Check sheet for the modelled part. Datum: model origin and axes. Units: mm. A direction names the side the tool comes from. Give positions to 0.01 mm unless a question says otherwise; leave off trailing zeros. Loops run counter-clockwise (first coordinate to the right, second up) from the corner with the lowest first, then second, coordinate; pieces in that order, holes last. Notation, with made-up numbers: (-21.5, 79) -> (11.5, 79) arc R8 cw to (11.5, 90) -> close; hole circle Ø6 at (22.5, 42.5). An arc over 180 degrees is marked (long way). Answer as CSV lines item,"result". Start each with the question number.
(1) Section check C-C on x = 7.5. Enter the section's corners in (y, z), plus the area to 3 significant figures.
(2) Material ranges on line 1 (Y direction, x = -11, z = 8); line 2 (X direction, y = 4.5, z = 4); line 3 (Z direction, x = 16, y = 2.25), recorded low to high. Write a range as from..to.
(3) Release check for a two-part mould opening along Y. For faces 1 (the face through (0, 3, 1)), 2 (the face through (0, -7.5, 27)), 3 (the face through (16.8, -7.64, 26.13)), 4 (the face through (0, 4, 0)) record: pulls with the +Y half, pulls with the -Y half, needs draft (parallel to the pull), parting line crosses it, or undercut.
(4) Gauge pin test, flat end, axial feed: pin 1 Ø4 at (x, y) = (-5.5, 6.5) entering from -Z. Record the tip position at first contact, or that the pin passes through.
(5) Section check D-D on y = 6.5. Enter the section's corners in (x, z).
(6) Section check A-A on z = 7. Enter the section's corners in (x, y), plus the area to 3 significant figures.
(7) Section check B-B on x = 1. Enter the section's corners in (y, z).
(8) Access from +Z, -Z, +X, -X, +Y, -Y to the whole of each face (thin tool, end or side, straight path). Record for faces 5 (the face through (2.2, 2, 0.5)), 6 (the face through (-16.84, -7.6, 26.13)), 7 (the face through (16.7, 0, 27)).
from build123d import *

# Parameters (mm, degrees)
F1_DEPTH = 53
F2_DEPTH = 1
F3_W     = 5
F3_H     = 4
F4_DEPTH = 53.001


with BuildPart() as f1:
    # F0 (on Top) → F1 (new body)
    with BuildSketch(Plane.XY):
        with BuildLine():
            Line((-14.7, -8.5), (14.7, -8.5))
            ThreePointArc((14.7, -8.5), (16.82132, -7.62132), (17.7, -5.5))
            Line((17.7, -5.5), (17.7, 5.5))
            ThreePointArc((17.7, 5.5), (16.82132, 7.62132), (14.7, 8.5))
            Line((14.7, 8.5), (-14.7, 8.5))
            ThreePointArc((-14.7, 8.5), (-16.82132, 7.62132), (-17.7, 5.5))
            Line((-17.7, 5.5), (-17.7, -5.5))
            ThreePointArc((-17.7, -5.5), (-16.82132, -7.62132), (-14.7, -8.5))
        make_face()
        with BuildLine():
            Line((-13.7, 7.5), (13.7, 7.5))
            ThreePointArc((13.7, 7.5), (15.82132, 6.62132), (16.7, 4.5))
            Line((16.7, 4.5), (16.7, -4.5))
            ThreePointArc((16.7, -4.5), (15.82132, -6.62132), (13.7, -7.5))
            Line((13.7, -7.5), (-13.7, -7.5))
            ThreePointArc((-13.7, -7.5), (-15.82132, -6.62132), (-16.7, -4.5))
            Line((-16.7, -4.5), (-16.7, 4.5))
            ThreePointArc((-16.7, 4.5), (-15.82132, 6.62132), (-13.7, 7.5))
        make_face(mode=Mode.SUBTRACT)
    extrude(amount=F1_DEPTH)

    # F0 (on Top) → F2 (join)
    with BuildSketch(Plane.XY):
        with BuildLine():
            ThreePointArc((16.7, 4.5), (15.82132, 6.62132), (13.7, 7.5))
            Line((13.7, 7.5), (-13.7, 7.5))
            ThreePointArc((-13.7, 7.5), (-15.82132, 6.62132), (-16.7, 4.5))
            Line((-16.7, 4.5), (-16.7, -4.5))
            ThreePointArc((-16.7, -4.5), (-15.82132, -6.62132), (-13.7, -7.5))
            Line((-13.7, -7.5), (13.7, -7.5))
            ThreePointArc((13.7, -7.5), (15.82132, -6.62132), (16.7, -4.5))
            Line((16.7, -4.5), (16.7, 4.5))
        make_face()
    extrude(amount=F2_DEPTH)

    # F3 (on face) → F4 (cut, through all)
    with BuildSketch(Plane(origin=(0, 0, 0), x_dir=(1, 0, 0), z_dir=(0, 0, -1))):
        with Locations((2.2, 0)):
            Rectangle(F3_W, F3_H)
    extrude(amount=-F4_DEPTH, mode=Mode.SUBTRACT)


solid = f1.part
Working result:
1,outline,"(-8.5, 0) -> (8.5, 0) -> (8.5, 53) -> (7.5, 53) -> (7.5, 1) -> (-7.5, 1) -> (-7.5, 53) -> (-8.5, 53) -> close"
1,area,"121 mm^2"
2,line 1,"y = -8.5..-7.5, 7.5..8.5"
2,line 2,"x = -17.7..-16.7, 16.7..17.7"
2,line 3,"z = 0..1"
3,face 1,"undercut"
3,face 2,"undercut"
3,face 3,"pulls with the -Y half"
3,face 4,"needs draft"
4,pin 1,"stops at z = 0"
5,outline,"(-17.53, 0) -> (17.53, 0) -> (17.53, 53) -> (15.94, 53) -> (15.94, 1) -> (-15.94, 1) -> (-15.94, 53) -> (-17.53, 53) -> close"
6,outline,"(-17.7, -5.5) arc R3 ccw to (-14.7, -8.5) -> (14.7, -8.5) arc R3 ccw to (17.7, -5.5) -> (17.7, 5.5) arc R3 ccw to (14.7, 8.5) -> (-14.7, 8.5) arc R3 ccw to (-17.7, 5.5) -> close; hole (-16.7, -4.5) arc R3 ccw to (-13.7, -7.5) -> (13.7, -7.5) arc R3 ccw to (16.7, -4.5) -> (16.7, 4.5) arc R3 ccw to (13.7, 7.5) -> (-13.7, 7.5) arc R3 ccw to (-16.7, 4.5) -> close"
6,area,"101 mm^2"
7,outline,"(-8.5, 0) -> (-2, 0) -> (-2, 1) -> (-7.5, 1) -> (-7.5, 53) -> (-8.5, 53) -> close; (2, 0) -> (8.5, 0) -> (8.5, 53) -> (7.5, 53) -> (7.5, 1) -> (2, 1) -> close"
8,face 5,"+Z, -Z"
8,face 6,"+Z, -Z, -X, -Y"
8,face 7,"+Z"
